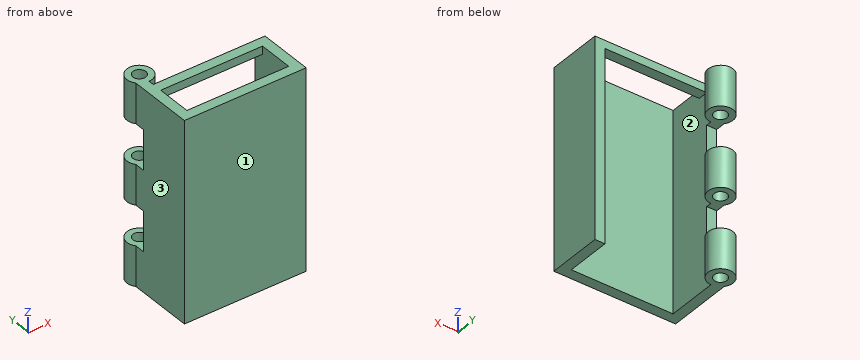
```python
from build123d import *

# Parameters (mm, degrees)
BATTERY_WALL_DEPTH  = 13.97
SKETCH1_4_W         = 25.908
SKETCH1_4_H         = 48.768
BATTERY_BASE_DEPTH  = 2.54
SKETCH3_W           = 25.908
SKETCH3_H           = 8.89
BATTERY_GAP_DEPTH   = 2.54
SKETCH4_R           = 1.651
BATTERY_HINGE_DEPTH = 10.16
LPATTERN1_COUNT     = 3
LPATTERN1_PITCH     = 20.32


with BuildPart() as part:
    # Sketch1 → battery-wall (new body)
    with BuildSketch(Plane(origin=(0, 0, 0), x_dir=(1, 0, 0), z_dir=(0, 1, 0))):
        Polygon((15.494, -26.416), (15.494, 24.384), (12.954, 24.384), (12.954, -24.384), (-12.954, -24.384), (-12.954, 24.384), (-15.494, 24.384), (-15.494, -26.416), align=None)
    extrude(amount=BATTERY_WALL_DEPTH)

    # Sketch1_4 → battery-base (add)
    with BuildSketch(Plane(origin=(0, 0, 0), x_dir=(1, 0, 0), z_dir=(0, 1, 0))):
        Rectangle(SKETCH1_4_W, SKETCH1_4_H)
    extrude(amount=BATTERY_BASE_DEPTH)

    # Sketch3 → battery-gap (cut)
    with BuildSketch(Plane.XY.offset(26.416)):
        with Locations((0, 6.985)):
            Rectangle(SKETCH3_W, SKETCH3_H)
    extrude(amount=-BATTERY_GAP_DEPTH, mode=Mode.SUBTRACT)

    # Sketch4 → battery-hinge (add)
    # profile 1 of 3: a face of its own
    with BuildSketch(Plane.XY.offset(26.416)):
        with BuildLine():
            Line((-15.494, 16.51), (-15.494, 13.97))
            Line((-15.494, 13.97), (-12.954, 13.97))
            Line((-12.954, 13.97), (-12.954, 15.366140824))
            ThreePointArc((-12.954, 15.366140824), (-14.356147146, 15.644630662), (-15.494, 16.51))
        make_face()
    # profile 2 of 3: a face of its own
    with BuildSketch(Plane.XY.offset(26.416)):
        with BuildLine():
            Line((-12.954, 16.51), (-15.494, 16.51))
            ThreePointArc((-15.494, 16.51), (-14.356147146, 15.644630662), (-12.954, 15.366140824))
            Line((-12.954, 15.366140824), (-12.954, 16.51))
        make_face()
    # profile 3 of 3: a face of its own
    with BuildSketch(Plane.XY.offset(26.416)):
        with BuildLine():
            ThreePointArc((-9.877425, 18.53961487), (-14.131457987, 21.52563443), (-15.494, 16.51))
            Line((-15.494, 16.51), (-12.954, 16.51))
            Line((-12.954, 16.51), (-12.954, 15.366140824))
            ThreePointArc((-12.954, 15.366140824), (-10.772828065, 16.329623283), (-9.877425, 18.53961487))
        make_face()
        with Locations((-13.052425, 18.53961487)):
            Circle(SKETCH4_R, mode=Mode.SUBTRACT)
    battery_hinge = extrude(amount=-BATTERY_HINGE_DEPTH)

    # LPattern1: battery-hinge ×3
    with Locations(*[(0, 0, -i * LPATTERN1_PITCH) for i in range(1, LPATTERN1_COUNT)]):
        add(battery_hinge)


solid = part.part
```
The listing builds one solid part. Answer for the finished solid, in the listing's coordinates (mm). Face numbers are marked on the shaded views. Give positions to 0.01 mm unless a question says otherwise; leave off trailing zeros. Order: outer loops, then holes, each group sorted by start corner. A loop starts at its lowest first (then second) coordinate and runs counter-clockwise, first axis right, second up. Notation, with made-up numbers: (72.5, 71.5) -> (92.5, 71.5) arc R14 cw to (92.5, 76.5) -> close; hole circle Ø9 at (33.5, 44). An arc over 180 degrees is marked (long way). One line per item, written item: value.
1) Find the intervals of material crossed by line 1 (X direction, y = 5, z = -1); line 2 (X direction, y = 14.25, z = 19.5); line 3 (Y direction, x = -5, z = 9.5), in increasing order.
Reported:
line 1: x = -15.49 to -12.95, 12.95 to 15.49
line 2: x = -15.49 to -12.95
line 3: y = 0 to 2.54
2) Find section D-D, the plane x = -12. Count the separate pieces of the cut face and the enclosed holes in it, plus the area to 3 significant figures.
Reported:
separate pieces: 8
enclosed holes: 0
area: 239 mm^2
3) Find section C-C, the plane y = 4.25. Determine the outline of the cut face in (x, z).
Reported:
outline: (-15.49, -24.38) -> (-12.95, -24.38) -> (-12.95, 26.42) -> (-15.49, 26.42) -> close; (12.95, -24.38) -> (15.49, -24.38) -> (15.49, 26.42) -> (12.95, 26.42) -> close
4) Flat-ended cylindrical pins translate along their axes: P1, Ø3, axis at x = 0.5, z = 18.5, coming from the +Y side; P2, Ø2, axis at x = 3.5, y = 12.5, coming from the -Z side; P3, Ø0.8, axis at x = -14, z = -11, coming from the +Y side. Find the tip coordinate at first contact, or state that the pin passes through.
Reported:
P1: stops at y = 2.54
P2: stops at z = 24.38
P3: stops at y = 13.97
5) Find section B-B, the plane z = -2. Determine the outline of the cut face in (x, y) (3 decimals).
Reported:
outline: (-15.494, 0) -> (15.494, 0) -> (15.494, 13.97) -> (12.954, 13.97) -> (12.954, 2.54) -> (-12.954, 2.54) -> (-12.954, 15.366) arc R3.175 ccw (long way) to (-15.494, 16.51) -> close; hole circle Ø3.302 at (-13.052, 18.54)
6) Find section A-A, the plane x = -2.5. Determine the outline of the cut face in (y, z), plus the area to 3 significant figures.
Reported:
outline: (0, -24.38) -> (2.54, -24.38) -> (2.54, 26.42) -> (0, 26.42) -> close; (11.43, 24.38) -> (13.97, 24.38) -> (13.97, 26.42) -> (11.43, 26.42) -> close
area: 134 mm^2
7) Determine the mould class of the marked faces 1, 2 and 3 for opening direction Y: pulls with the +Y half, pulls with the -Y half, needs draft (parallel to the pull), parting line crosses it, or undercut.
Reported:
face 1: pulls with the -Y half
face 2: undercut
face 3: needs draft
